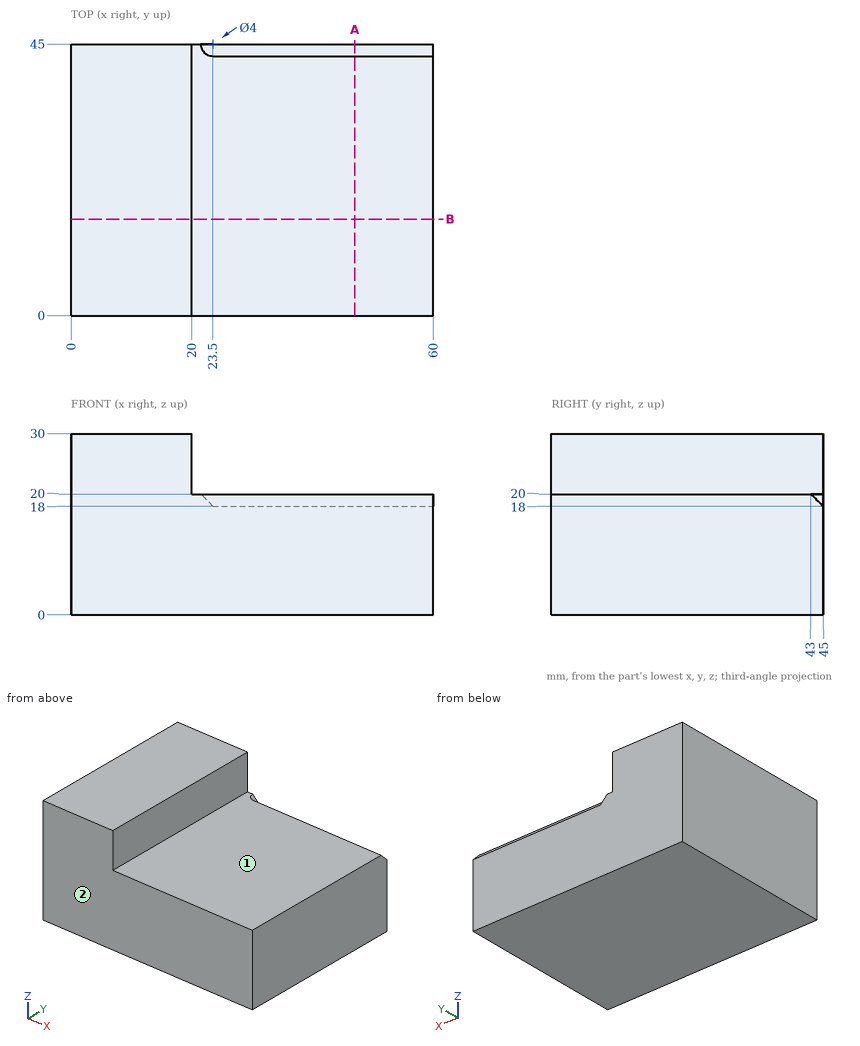
Input: dimensioned drawing with shaded views. Units: mm. Origin: part minimum x, y, z. A direction names the side the tool comes from. Coordinates: 2 decimals unless noted, no trailing zeros. Write each loop counter-clockwise with the first axis right and the second up, starting at its lowest first coordinate (ties: lowest second). Pieces come first, ordered by that corner, then holes. Notation, with made-up numbers: (70.5, -7) -> (99.5, -7) arc R13 ccw to (99.5, 8) -> close; hole circle Ø11 at (10.25, -2). An arc over 180 degrees is marked (long way). Return JSON: item names as keys, results as strings. Group by question number.
1) Ray query, line 1 along Z through (x, y) = (57, 11.5); line 2 along Y through (x, z) = (33.5, 19.25). Return the intervals inside material, ascending.
2) Section query B-B, the plane y = 16. Return loops of the section in (x, z).
3) Section query A-A, the plane x = 47. Return loops of the section in (y, z).
4) Contact query for flat-ended pins moving along their axis: P1, Ø1, axis at x = 41, y = 23.5, coming from the +Z side; P2, Ø1.5, axis at x = 45.5, z = 19.5, coming from the +Y side; P3, Ø5, axis at y = 13.5, z = 24.5, coming from the +X side. Output: stop coordinate, or through.
5) Set-up query: the marked faces 1 and 2. Return all of +Z, -Z, +X, -X, +Y, -Y with unobstructed straight access to the full face (end or side cutting, diameter ignored); none if empty.
From the geometry:
{
 "1": {"line 1": "0 to 20", "line 2": "0 to 43.75"},
 "2": {"outline": "(0, 0) -> (60, 0) -> (60, 20) -> (20, 20) -> (20, 30) -> (0, 30) -> close"},
 "3": {"outline": "(0, 0) -> (45, 0) -> (45, 18) -> (43, 20) -> (0, 20) -> close"},
 "4": {"P1": "z = 20", "P2": "y = 44.25", "P3": "x = 20"},
 "5": {"face 1": "+Z, +X, +Y, -Y", "face 2": "+Z, -Z, +X, -X, -Y"}
}
